Part model, mm, in its own coordinate system. A direction names the side the tool comes from. Round coordinates to 2 decimals unless told otherwise and drop trailing zeros. Order: outer loops, then holes, each group sorted by start corner. A loop starts at its lowest first (then second) coordinate and runs counter-clockwise, first axis right, second up. Notation, with made-up numbers: (69.5, 44.5) - (101.5, 44.5) arc R12 cw to (101.5, 62.5) - close; hole circle Ø3 at (-13.75, -15). An arc over 180 degrees is marked (long way). Answer as a JSON object with one key per item and string values.
```python
from build123d import *

# Parameters (mm, degrees)
F0_W     = 32.73212
F0_H     = 2.54
F0_W_2   = 11.01766
F1_DEPTH = 1.27
F2_W     = 32.73212
F2_H     = 5.08
F2_W_2   = 11.01766
F3_DEPTH = 7.7089
F4_W     = 97.79
F4_H     = 50.165
F5_DEPTH = 3.175
F6_R     = 1.27


with BuildPart() as f1:
    # F0 (on Top) → F1 (new body)
    with BuildSketch(Plane.XY):
        Polygon((13.35448, 42.545), (13.35448, 45.085), (0, 45.085), (0, 0), (12.98618, 0), (12.98618, 2.54), (2.54, 2.54), (2.54, 42.545), align=None)
        Polygon((73.68624, 42.545), (90.17, 42.545), (90.17, 2.54), (67.35402, 2.54), (67.35402, 0), (92.71, 0), (92.71, 45.085), (73.68624, 45.085), align=None)
        with Locations((47.3202, 43.815)):
            Rectangle(F0_W, F0_H)
        with Locations((43.84421, 1.27)):
            Rectangle(F0_W_2, F0_H)
    extrude(amount=F1_DEPTH)

    # F2 (on face) → F3 (join)
    with BuildSketch(Plane.XY.offset(1.27)):
        Polygon((12.98618, 2.54), (2.54, 2.54), (2.54, 42.545), (13.35448, 42.545), (13.35448, 47.625), (-2.54, 47.625), (-2.54, -2.54), (12.98618, -2.54), align=None)
        Polygon((90.17, 42.545), (90.17, 2.54), (67.35402, 2.54), (67.35402, -2.54), (95.25, -2.54), (95.25, 47.625), (73.68624, 47.625), (73.68624, 42.545), align=None)
        with Locations((47.3202, 45.085)):
            Rectangle(F2_W, F2_H)
        with Locations((43.84421, 0)):
            Rectangle(F2_W_2, F2_H)
    extrude(amount=F3_DEPTH)

    # F4 (on face) → F5 (join)
    with BuildSketch(Plane.XY.offset(8.9789)):
        with Locations((46.355, 22.5425)):
            Rectangle(F4_W, F4_H)
    extrude(amount=F5_DEPTH)

    # F6
    f6_edges = [f1.edges().sort_by_distance(p)[0] for p in [
        (95.25, -2.54, 6.71195),
        (-2.54, -2.54, 6.71195),
        (95.25, 47.625, 6.71195),
        (-2.54, 47.625, 6.71195),
        (-2.54, 22.5425, 12.1539),
        (46.355, -2.54, 12.1539),
        (95.25, 22.5425, 12.1539),
        (46.355, 47.625, 12.1539),
    ]]
    fillet(f6_edges, radius=F6_R)


solid = f1.part
```
Item 1: Cut at D-D (y = 3.5). Write the cut outline in (x, z), plus the area to 3 significant figures.
Taken from the geometry:
{"outline": "(-2.54, 1.27) - (0, 1.27) - (0, 0) - (2.54, 0) - (2.54, 8.98) - (90.17, 8.98) - (90.17, 0) - (92.71, 0) - (92.71, 1.27) - (95.25, 1.27) - (95.25, 10.88) arc R1.27 ccw to (93.98, 12.15) - (-1.27, 12.15) arc R1.27 ccw to (-2.54, 10.88) - close", "area": "395 mm2"}
Item 2: Cut at A-A (z = 5.25). Write the cut outline in (x, y) (3 decimals).
Taken from the geometry:
{"outline": "(-2.54, -1.27) arc R1.27 ccw to (-1.27, -2.54) - (12.986, -2.54) - (12.986, 2.54) - (2.54, 2.54) - (2.54, 42.545) - (13.354, 42.545) - (13.354, 47.625) - (-1.27, 47.625) arc R1.27 ccw to (-2.54, 46.355) - close; (30.954, 42.545) - (63.686, 42.545) - (63.686, 47.625) - (30.954, 47.625) - close; (38.335, -2.54) - (49.353, -2.54) - (49.353, 2.54) - (38.335, 2.54) - close; (67.354, -2.54) - (93.98, -2.54) arc R1.27 ccw to (95.25, -1.27) - (95.25, 46.355) arc R1.27 ccw to (93.98, 47.625) - (73.686, 47.625) - (73.686, 42.545) - (90.17, 42.545) - (90.17, 2.54) - (67.354, 2.54) - close"}
Item 3: Tool access for faces 1 (the flat face through (38.335, 0, 4)), 2 (the flat face through (63.686, 45, 4)), 3 (the flat face through (73.686, 45, 4)): list every direction of +Z, -Z, +X, -X, +Y, -Y with a clear straight run to the whole face (end or side of a thin tool).
Taken from the geometry:
{"face 1": "-Z, -Y", "face 2": "-Z, +Y, -Y", "face 3": "-Z, +Y"}
Item 4: Probe L1, parallel to X at y = 43.5, z = 8.25; L2, parallel to X at y = 2, z = 1.75; L3, parallel to X at y = 24, z = 7.75. List the from-to ranges inside material, lowest first. Write a range as from..to.
Taken from the geometry:
{"L1": "-2.54..13.35, 30.95..63.69, 73.69..95.25", "L2": "-2.54..12.99, 38.34..49.35, 67.35..95.25", "L3": "-2.54..2.54, 90.17..95.25"}
Item 5: Two-plate mould, pull along Y, no slides. Class faces 4 (the flat face through (91, 24, 0)), 5 (the flat face through (8, 42.545, 4)): pulls with the +Y half, pulls with the -Y half, needs draft (parallel to the pull), parting line crosses it, or undercut.
Taken from the geometry:
{"face 4": "needs draft", "face 5": "undercut"}
Item 6: Cut at B-B (x = 11.5). Write the cut outline in (y, z) (3 decimals), plus the area to 3 significant figures.
Taken from the geometry:
{"outline": "(-2.54, 1.27) - (0, 1.27) - (0, 0) - (2.54, 0) - (2.54, 8.979) - (42.545, 8.979) - (42.545, 0) - (45.085, 0) - (45.085, 1.27) - (47.625, 1.27) - (47.625, 10.884) arc R1.27 ccw to (46.355, 12.154) - (-1.27, 12.154) arc R1.27 ccw to (-2.54, 10.884) - close", "area": "243 mm2"}
Item 7: Cut at C-C (y = 44). Write the cut outline in (x, z), plus the area to 3 significant figures.
Taken from the geometry:
{"outline": "(-2.54, 1.27) - (0, 1.27) - (0, 0) - (13.35, 0) - (13.35, 8.98) - (30.95, 8.98) - (30.95, 0) - (63.69, 0) - (63.69, 8.98) - (73.69, 8.98) - (73.69, 0) - (92.71, 0) - (92.71, 1.27) - (95.25, 1.27) - (95.25, 10.88) arc R1.27 ccw to (93.98, 12.15) - (-1.27, 12.15) arc R1.27 ccw to (-2.54, 10.88) - close", "area": "934 mm2"}
Item 8: Drop flat-ended pins along their axis: P1, Ø1.3, axis at x = 45, y = -1.5, coming from the -Z side; P2, Ø3, axis at x = 53, y = 18, coming from the -Z side; P3, Ø8.5, axis at x = 86, y = 10, coming from the -Z side; P4, Ø1.4, axis at x = 53, z = 0.5, coming from the +Y side (3 decimals). Give the stop position or say it passes through.
Taken from the geometry:
{"P1": "z = 1.27", "P2": "z = 8.98", "P3": "z = 0", "P4": "y = 45.085"}
